Work out the finished part from the listing and answer in its coordinate system (mm). Coordinates: 2 decimals unless noted, no trailing zeros. Order: outer loops, then holes, each group sorted by start corner. A loop starts at its lowest first (then second) coordinate and runs counter-clockwise, first axis right, second up. Notation, with made-up numbers: (68.5, -21) -> (94.5, -21) arc R8 cw to (94.5, -11) -> close; hole circle Ø8 at (-39, -8.5). An arc over 180 degrees is marked (long way). Use one line per item in the form item = value.
from build123d import *

# Parameters (mm, degrees)
F0_W           = 171
F0_H           = 133
F1_DEPTH       = 18
F4_D           = 4
F4_CSINK_D     = 8.2
F4_CSINK_ANGLE = 90
F5_D           = 4
F5_CSINK_D     = 8.2
F5_CSINK_ANGLE = 90
F7_D           = 4
F7_CSINK_D     = 8.2
F7_CSINK_ANGLE = 90


# Not quite as in the source:
# - a feature of the source that left no trace in its solid (it failed there, or was rolled back) is left out


with BuildPart() as f1:
    # F0 (on Front) → F1 (new body)
    with BuildSketch(Plane.XZ):
        Rectangle(F0_W, F0_H)
    extrude(amount=F1_DEPTH)

    # F4 (through all)
    with Locations(Plane.XZ.offset(18)):
        with Locations((0, -39.5)):
            CounterSinkHole(F4_D / 2, F4_CSINK_D / 2, counter_sink_angle=F4_CSINK_ANGLE)

    # F5 (through all)
    with Locations(Plane.XZ.offset(18)):
        with Locations((-76.5, -39.5), (76.5, -39.5)):
            CounterSinkHole(F5_D / 2, F5_CSINK_D / 2, counter_sink_angle=F5_CSINK_ANGLE)

    # F7 (through all)
    with Locations(Plane.XZ.offset(18)):
        with Locations((-76.5, 39.5), (76.5, 39.5)):
            CounterSinkHole(F7_D / 2, F7_CSINK_D / 2, counter_sink_angle=F7_CSINK_ANGLE)


solid = f1.part
(1) Section C-C on x = -76.5 is taken. Write down the section's boundary in (y, z), plus the area to 3 significant figures.
Data:
outline = (-18, -66.5) -> (0, -66.5) -> (0, -41.5) -> (-15.9, -41.5) -> (-18, -43.6) -> close; (-18, -35.4) -> (-15.9, -37.5) -> (0, -37.5) -> (0, 37.5) -> (-15.9, 37.5) -> (-18, 35.4) -> close; (-18, 43.6) -> (-15.9, 41.5) -> (0, 41.5) -> (0, 66.5) -> (-18, 66.5) -> close
area = 2,240 mm²
(2) Section B-B on x = 0 is taken. Write down the section's boundary in (y, z).
Data:
outline = (-18, -66.5) -> (0, -66.5) -> (0, -41.5) -> (-15.9, -41.5) -> (-18, -43.6) -> close; (-18, -35.4) -> (-15.9, -37.5) -> (0, -37.5) -> (0, 66.5) -> (-18, 66.5) -> close
(3) The mould has two halves that part along Z. Classify faces 1 (the cylindrical face through (75.577, -7.839, -41.274)), 2 (the flat face through (-1, 0, 1)), 3 (the flat face through (-1, -9, -66.5)): released by +Z, released by -Z, zero draft, split by the parting line, or undercut.
Data:
face_1 = undercut
face_2 = zero draft
face_3 = released by -Z
(4) Straight lines are drawn through the part: line 1 along X through (y, z) = (-7, 39.5); line 2 along Z through (x, y) = (76.5, -6.25); line 3 along X through (y, z) = (-8, -39.5). For each, find the intervals that lie inside material, in ascending order.
Data:
line_1 = -85.5 to -78.5, -74.5 to 74.5, 78.5 to 85.5
line_2 = -66.5 to -41.5, -37.5 to 37.5, 41.5 to 66.5
line_3 = -85.5 to -78.5, -74.5 to -2, 2 to 74.5, 78.5 to 85.5
(5) Section A-A on z = -39.5 is taken. Write down the section's boundary in (x, y).
Data:
outline = (-85.5, -18) -> (-80.6, -18) -> (-78.5, -15.9) -> (-78.5, 0) -> (-85.5, 0) -> close; (-74.5, -15.9) -> (-72.4, -18) -> (-4.1, -18) -> (-2, -15.9) -> (-2, 0) -> (-74.5, 0) -> close; (2, -15.9) -> (4.1, -18) -> (72.4, -18) -> (74.5, -15.9) -> (74.5, 0) -> (2, 0) -> close; (78.5, -15.9) -> (80.6, -18) -> (85.5, -18) -> (85.5, 0) -> (78.5, 0) -> close
(6) Section D-D on z = 39.5 is taken. Write down the section's boundary in (x, y).
Data:
outline = (-85.5, -18) -> (-80.6, -18) -> (-78.5, -15.9) -> (-78.5, 0) -> (-85.5, 0) -> close; (-74.5, -15.9) -> (-72.4, -18) -> (72.4, -18) -> (74.5, -15.9) -> (74.5, 0) -> (-74.5, 0) -> close; (78.5, -15.9) -> (80.6, -18) -> (85.5, -18) -> (85.5, 0) -> (78.5, 0) -> close
(7) This flat-tipped pin is pushed along its axis until it touches: P1, Ø5, axis at x = -76.5, z = 39.5, coming from the +Y side. Where does it stop, or does it pass through?
Data:
P1 = 0
